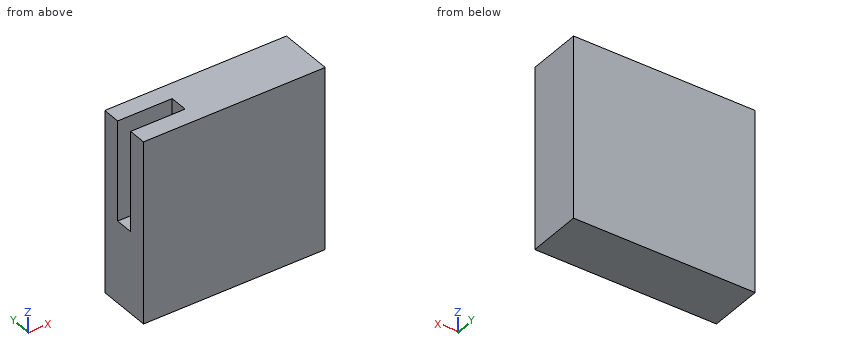
Autodesk Inventor part; units mm, degrees
ref_plane "YZ Plane" through (0, 0, 0) normal (1, 0, 0) x (0, 1, 0)
ref_plane "XZ Plane" through (0, 0, 0) normal (0, 1, 0) x (-1, 0, 0)
ref_plane "XY Plane" through (0, 0, 0) normal (0, 0, 1) x (1, 0, 0)
sketch "Sketch1" plane through (0, 0, 0) normal (0, 1, 0) x (-1, 0, 0)
  line L0 (10, 10) -> (-10, 10)
  line L1 (-10, 10) -> (-10, -10)
  line L2 (-10, -10) -> (10, -10)
  line L3 (10, -10) -> (10, 10)
  line L4 (10, 10) -> (-10, -10) construction
  line L5 (-10, 10) -> (10, -10) construction
  point P0 (0, 0)
  dimension "d0" = 20
  dimension "d1" = 20
extrude "Extrusion1" add sketch "Sketch1" along normal blind 6
sketch "Sketch2" plane through (-10, 0, 10) normal (0, 0, 1) x (1, 0, 0)
  line L0 (0, 0) -> (0, 6)
  line L1 (0, 4) -> (6, 4)
  line L2 (6, 4) -> (6, 2)
  line L3 (6, 2) -> (0, 2)
  line L4 (0, 2) -> (0, 4)
  line L5 (0, 0) -> (20, 0)
  point P0 (10, 0)
  point P1 (0, 2)
  dimension "d4" = 6
  dimension "d5" = 2
  dimension "d6" = 2
extrude "Extrusion2" cut sketch "Sketch2" against normal blind 3
sketch "Sketch3" plane through (-10, 0, -10) normal (-1, 0, 0) x (0, 0, 1)
  line L0 (20, 4) -> (17, 4)
  line L1 (20, 4) -> (9, 4)
  line L2 (9, 4) -> (9, 2)
  line L3 (9, 2) -> (20, 2)
  line L4 (20, 2) -> (20, 4)
  point P0 (10, 0)
  dimension "d9" = 11
  dimension "d10" = 2
extrude "Extrusion3" cut sketch "Sketch3" against normal blind 3
properties part number "Bracket Lifter Motor_3DPrint"
The model under review builds one solid part; all positions refer to its coordinate system, in mm. Round coordinates to 2 decimals unless told otherwise and drop trailing zeros. Order: outer loops, then holes, each group sorted by start corner. A loop starts at its lowest first (then second) coordinate and runs counter-clockwise, first axis right, second up. Notation, with made-up numbers: M 80.5,83 L 93.5,83 A13 cw 93.5,93 Z; hole C -26,76.25 d11. An arc over 180 degrees is marked long. Use a Markdown table: item, result.
1) Consider section B-B (z = 6). Write out the cut boundary in (x, y).
Report:
| item | result |
|---|---|
| outline | M -10,0 L 10,0 L 10,6 L -10,6 L -10,4 L -7,4 L -7,2 L -10,2 Z |
2) Insertion check: pin 1 (10 mm diameter, centred on x = -3.5, z = 8, fed in from -Y); pin 2 (1 mm diameter, centred on x = -5.5, y = 3, fed in from +Z); pin 3 (0.6 mm diameter, centred on y = 3, z = 9, fed in from -X). Each pin has a flat end and moves straight along its axis. Give the tip position at first contact, or say it passes through.
Report:
| item | result |
|---|---|
| pin 1 | y = 0 |
| pin 2 | z = 7 |
| pin 3 | x = -4 |
3) Wall thickness on line 1 along Y through (x, z) = (-9, 2); line 2 along X through (y, z) = (3.5, 1.5); line 3 along Z through (x, y) = (-6.75, 2.2): over which ranges is each line inside the solid? List them lowest first. Write a range as [from, to].
Report:
| item | result |
|---|---|
| line 1 | [0, 2], [4, 6] |
| line 2 | [-7, 10] |
| line 3 | [-10, 7] |
4) Consider section A-A (x = -8.5). Write out the cut boundary in (y, z), then the cut area to 3 significant figures.
Report:
| item | result |
|---|---|
| outline | M 0,-10 L 6,-10 L 6,10 L 4,10 L 4,-1 L 2,-1 L 2,10 L 0,10 Z |
| area | 98.0 mm^2 |
